Verification items for the finished model (mm, model axes). Face numbers are marked on the shaded views. A direction names the side the tool comes from. Round coordinates to 2 decimals unless told otherwise and drop trailing zeros. Write each loop counter-clockwise with the first axis right and the second up, starting at its lowest first coordinate (ties: lowest second). Pieces come first, ordered by that corner, then holes. Notation, with made-up numbers: M -18.75,87.25 L 36.25,87.25 A29 cw 36.25,120.25 Z; hole C -13.75,-19.5 d9. An arc over 180 degrees is marked long. One line per question, with ' | ' between items. Start each with the question number.
Q1. Thickness scan on line 1 along Y through (x, z) = (0, 9.45); line 2 along Y through (x, z) = (0, 1.6); line 3 along Z through (x, y) = (9, -5.5). Record the ranges inside material, lowest first. Write a range as from..to.
Q2. Release check for a two-part mould opening along X. For the marked faces 4, 5 and 6 record: released by +X, released by -X, zero draft, split by the parting line, or undercut.
Q3. Cross-section at B-B (y = 12.5). Record the boundary of the cut face in (x, z).
Q4. Gauge pin test, flat ends, axial feed: pin 1 (22.5 mm diameter, centred on x = 0, y = 0, fed in from -Z); pin 2 (10 mm diameter, centred on x = -4, y = -5, fed in from +Z); pin 3 (4 mm diameter, centred on y = -21.5, z = 7, fed in from +X); pin 4 (3 mm diameter, centred on y = 8, z = 7, fed in from -X). Record the tip position at first contact, or that the pin passes through.
Q5. Cross-section at A-A (y = 3). Record the boundary of the cut face in (x, z).
Q6. Tool access check on the marked faces 1, 2 and 3. Record the directions out of +Z, -Z, +X, -X, +Y, -Y that give a thin tool (end or side, any length) a straight path to the whole face; none if there is none.
from build123d import *

# Parameters (mm, degrees)
SKETCH1_R           = 8
SKETCH1_R_2         = 7
BOSS_EXTRUDE1_DEPTH = 3.43
SKETCH2_R           = 14.5
SKETCH2_R_2         = 4.625
BOSS_EXTRUDE2_DEPTH = 2
SKETCH3_R           = 11.75
SKETCH3_R_2         = 1.35
BOSS_EXTRUDE3_DEPTH = 3.5
BOSS_EXTRUDE4_START = 2
SKETCH4_R           = 1.35
BOSS_EXTRUDE4_DEPTH = 2
CUT_EXTRUDE1_START  = -3.5
CUT_EXTRUDE1_DEPTH  = 3.5
FILLET1_R           = 2
SKETCH8_R           = 2.5
SKETCH8_R_2         = 1.35
BOSS_EXTRUDE6_DEPTH = 1.5


# Read off the part's stored shape, not the designer's step: Cut-Extrude1
with BuildPart() as part:
    # Sketch1 → Boss-Extrude1 (new body)
    with BuildSketch(Plane.XY):
        with Locations(Location((0, 0, 0), (0, 0, 180))):
            Circle(SKETCH1_R)
        with Locations(Location((0, 0, 0), (0, 0, 180))):
            Circle(SKETCH1_R_2, mode=Mode.SUBTRACT)
    extrude(amount=BOSS_EXTRUDE1_DEPTH)

    # Sketch2 → Boss-Extrude2 (add)
    with BuildSketch(Plane.XY.offset(3.43)):
        Circle(SKETCH2_R)
        Circle(SKETCH2_R_2, mode=Mode.SUBTRACT)
    extrude(amount=BOSS_EXTRUDE2_DEPTH)

    # Sketch3 → Boss-Extrude3 (add)
    with BuildSketch(Plane.XY.offset(5.43)):
        with BuildLine():
            Line((3.75, -24), (3.75, -20.277758752))
            ThreePointArc((3.75, -20.277758752), (4.914773659, -15.593874092), (8.137755102, -12.001122527))
            ThreePointArc((8.137755102, -12.001122527), (10.253048327, 10.253048327), (-12.001122527, 8.137755102))
            ThreePointArc((-12.001122527, 8.137755102), (-15.593874092, 4.914773659), (-20.277758752, 3.75))
            Line((-20.277758752, 3.75), (-27, 3.75))
            ThreePointArc((-27, 3.75), (-29.651650429, 2.651650429), (-30.75, 0))
            add(Edge.make_bspline(
                [(-30.75, 0), (-30.75, -27.75), (0, -27.75)],
                knots=[0, 0, 0, 1.570796327, 1.570796327, 1.570796327], degree=2, weights=[1, 0.707106781, 1]))
            ThreePointArc((0, -27.75), (2.651650429, -26.651650429), (3.75, -24))
        make_face()
        Circle(SKETCH3_R, mode=Mode.SUBTRACT)
        with Locations((0, -24)):
            Circle(SKETCH3_R_2, mode=Mode.SUBTRACT)
        with Locations((-27, 0)):
            Circle(SKETCH3_R_2, mode=Mode.SUBTRACT)
    extrude(amount=BOSS_EXTRUDE3_DEPTH)

    # Sketch4 → Boss-Extrude4 (add)
    with BuildSketch(Plane(origin=(0, 0, 5.43), x_dir=(-1, 0, 0), z_dir=(0, 0, -1)).offset(BOSS_EXTRUDE4_START)):
        with BuildLine():
            Line((-3.75, -20.277758752), (-3.75, -24))
            ThreePointArc((-3.75, -24), (-2.651650429, -26.651650429), (0, -27.75))
            add(Edge.make_bspline(
                [(0, -27.75), (30.75, -27.75), (30.75, 0)],
                knots=[4.71238898, 4.71238898, 4.71238898, 6.283185307, 6.283185307, 6.283185307], degree=2, weights=[1, 0.707106781, 1]))
            ThreePointArc((30.75, 0), (29.651650429, 2.651650429), (27, 3.75))
            Line((27, 3.75), (20.277758752, 3.75))
            ThreePointArc((20.277758752, 3.75), (15.593874092, 4.914773659), (12.001122527, 8.137755102))
            ThreePointArc((12.001122527, 8.137755102), (10.253048327, -10.253048327), (-8.137755102, -12.001122527))
            ThreePointArc((-8.137755102, -12.001122527), (-4.914773659, -15.593874092), (-3.75, -20.277758752))
        make_face()
        with Locations(Location((27, 0, 0), (0, 0, 180))):
            Circle(SKETCH4_R, mode=Mode.SUBTRACT)
        with Locations(Location((0, -24, 0), (0, 0, 180))):
            Circle(SKETCH4_R, mode=Mode.SUBTRACT)
    extrude(amount=-BOSS_EXTRUDE4_DEPTH)

    # Cut-Extrude1 outline → Cut-Extrude1 (cut)
    with BuildSketch(Plane.XY.offset(8.93).offset(CUT_EXTRUDE1_START)):
        with BuildLine():
            ThreePointArc((-23.887668919, -2.091864059), (-25.551843779, -3.459095772), (-27.693722308, -3.685274665))
            add(Edge.make_bspline(
                [(-27.693722308, -3.685274665), (-27.362240175, -5.665830378), (-25.799154504, -10.759842679), (-20.433371513, -18.029392928), (-12.653019422, -22.727558912), (-6.72944223, -24.348951045), (-4.285685075, -24.711452028), (-3.667038232, -24.784430116)],
                knots=[0.149690792, 0.149690792, 0.149690792, 0.149690792, 0.392699082, 0.785398163, 1.178097245, 1.374446786, 1.440624357, 1.440624357, 1.440624357, 1.440624357], degree=3))
            ThreePointArc((-3.667038232, -24.784430116), (-3.522792072, -22.714528875), (-2.300027155, -21.038180444))
            ThreePointArc((-2.300027155, -21.038180444), (-0.83329357, -17.083388646), (-3.725629572, -14.013196791))
            ThreePointArc((-3.725629572, -14.013196791), (-10.247441141, -10.258652449), (-14.009114583, -3.740950226))
            ThreePointArc((-14.009114583, -3.740950226), (-18.417300739, 0.264998128), (-23.887668919, -2.091864059))
        make_face()
    extrude(amount=CUT_EXTRUDE1_DEPTH, mode=Mode.SUBTRACT)

    # Fillet1
    fillet1_edges = [part.edges().sort_by_distance(p)[0] for p in [
        (-3.667038232, -24.784430116, 7.18),
        (-27.693722308, -3.685274665, 7.18),
    ]]
    fillet(fillet1_edges, radius=FILLET1_R)

    # Sketch8 → Boss-Extrude6 (add)
    with BuildSketch(Plane.XY.offset(8.93)):
        with Locations((0, -24)):
            Circle(SKETCH8_R)
        with Locations((0, -24)):
            Circle(SKETCH8_R_2, mode=Mode.SUBTRACT)
    extrude(amount=BOSS_EXTRUDE6_DEPTH)


solid = part.part
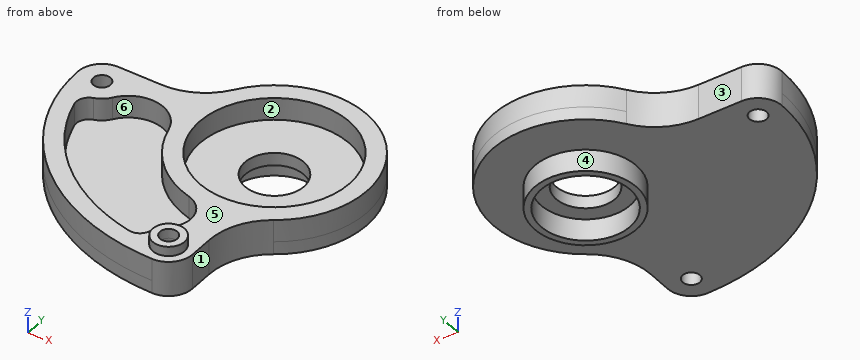
Determined:
1) line 1: y = -26.5..-25.35, -22.65..-21.5 | line 2: y = -8..-7, 7..8 | line 3: z = 3.43..5.43
2) face 4: split by the parting line | face 5: zero draft | face 6: undercut
3) outline: M -7.35,3.43 L 7.35,3.43 L 7.35,8.93 L -7.35,8.93 Z
4) pin 1: stops at z = 0 | pin 2: stops at z = 5.43 | pin 3: stops at x = 3.78 | pin 4: stops at x = -13.39
5) outline: M -29.25,3.43 L -7.42,3.43 L -7.42,0 L -6.32,0 L -6.32,3.43 L -3.52,3.43 L -3.52,5.43 L -11.36,5.43 L -11.36,8.93 L -29.25,8.93 Z; M 3.52,3.43 L 6.32,3.43 L 6.32,0 L 7.42,0 L 7.42,3.43 L 14.19,3.43 L 14.19,8.93 L 11.36,8.93 L 11.36,5.43 L 3.52,5.43 Z
6) face 1: +Z, -Z, +X, -Y | face 2: +Z | face 3: +Z, -Z, -X, +Y
